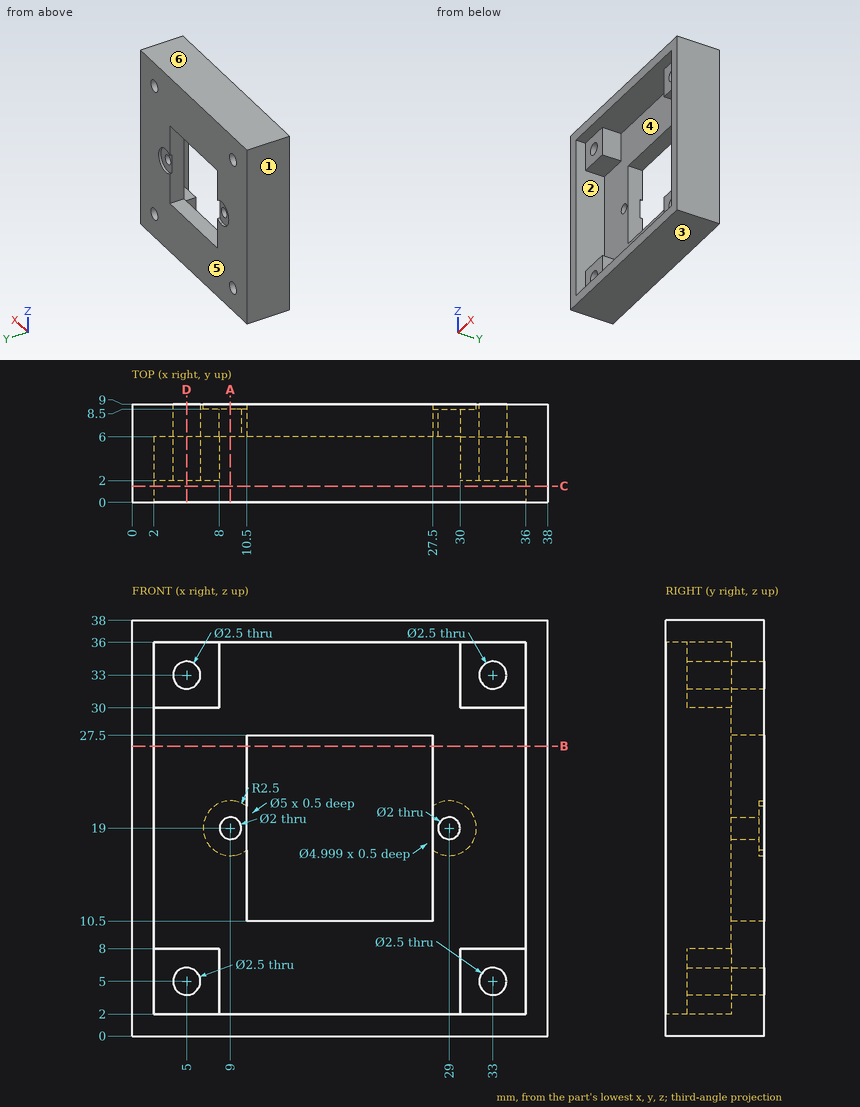
For this review, use the dimensioned drawing (mm, ordinates from the lowest corner) and the shaded views. A direction names the side the tool comes from. Coordinates: 2 decimals unless noted, no trailing zeros. Loops run counter-clockwise (first coordinate to the right, second up) from the corner with the lowest first, then second, coordinate; pieces in that order, holes last. Notation, with made-up numbers: (87.5, 5) -> (100.5, 5) arc R19 ccw to (100.5, 27) -> close; hole circle Ø10 at (19.5, -17). An arc over 180 degrees is marked (long way). Use a Markdown table: item, result. Add a question column.
Item 1: We need section C-C, the plane y = 1.5. Write out the cut boundary in (x, z), and give its area (3 significant figures).
Item 2: Clearance check with flat-ended pins moving along their axes: P1, Ø5, axis at x = 32.5, z = 26, coming from the -Y side; P2, Ø2, axis at x = 33, z = 5, coming from the +Y side; P3, Ø1.8, axis at x = 4.5, z = 33.5, coming from the -Y side. State where each tip first meets the part, or that it passes through.
Item 3: Wall thickness on L1, parallel to X at y = 4.75, z = 33; L2, parallel to X at y = 4.75, z = 21.5: over which ranges is each line inside the solid? List them lowest first. Write a range as from..to.
Item 4: Machinability: for the marked faces 1 and 2, which of the approach directions +Z, -Z, +X, -X, +Y, -Y give a long, thin tool a straight path to every point of the face, cutting with its end or side? Answer none if there is none.
Item 5: We need section B-B, the plane z = 26.5. Write out the cut boundary in (x, y).
Item 6: We need section D-D, the plane x = 5. Write out the cut boundary in (y, z).
Item 7: We need section A-A, the plane x = 9. Write out the cut boundary in (y, z).
Item 8: The part is to be moulded in two halves that separate along Z. For the marked faces 3, 4, 5 and 6, say which applies: +Z half, -Z half, draft (parallel to the pull), parting line (faces both ways), or undercut.
Numbers:
| question | item | result |
|---|---|---|
| 1 | outline | (0, 0) -> (38, 0) -> (38, 38) -> (0, 38) -> close; hole (2, 2) -> (36, 2) -> (36, 36) -> (2, 36) -> close |
| 1 | area | 288 mm^2 |
| 2 | P1 | stops at y = 6 |
| 2 | P2 | passes through |
| 2 | P3 | stops at y = 2 |
| 3 | L1 | x = 0..3.75, 6.25..8, 30..31.75, 34.25..38 |
| 3 | L2 | x = 0..2, 36..38 |
| 4 | face 1 | +Z, -Z, -X, +Y, -Y |
| 4 | face 2 | -Y |
| 5 | outline | (0, 0) -> (2, 0) -> (2, 6) -> (10.5, 6) -> (10.5, 9) -> (0, 9) -> close; (27.5, 6) -> (36, 6) -> (36, 0) -> (38, 0) -> (38, 9) -> (27.5, 9) -> close |
| 6 | outline | (0, 0) -> (9, 0) -> (9, 3.75) -> (2, 3.75) -> (2, 2) -> (0, 2) -> close; (0, 36) -> (2, 36) -> (2, 34.25) -> (9, 34.25) -> (9, 38) -> (0, 38) -> close; (2, 6.25) -> (9, 6.25) -> (9, 31.75) -> (2, 31.75) -> (2, 30) -> (6, 30) -> (6, 8) -> (2, 8) -> close |
| 7 | outline | (0, 0) -> (9, 0) -> (9, 16.5) -> (8.5, 16.5) -> (8.5, 18) -> (6, 18) -> (6, 2) -> (0, 2) -> close; (0, 36) -> (6, 36) -> (6, 20) -> (8.5, 20) -> (8.5, 21.5) -> (9, 21.5) -> (9, 38) -> (0, 38) -> close |
| 8 | face 3 | -Z half |
| 8 | face 4 | undercut |
| 8 | face 5 | draft |
| 8 | face 6 | +Z half |
